from build123d import *

# Parameters (mm, degrees)
F0_R     = 7
F1_DEPTH = 25.4
F2_R     = 3.81
F3_DEPTH = 21.59
F4_R     = 7
F4_R_2   = 5.715
F5_DEPTH = 20.32
F6_W     = 2.794
F6_H     = 2.54
F7_DEPTH = 25.4
F8_R     = 0.9525
F9_DEPTH = 5.08


with BuildPart() as f1:
    # F0 (on Top) → F1 (new body)
    with BuildSketch(Plane.XY):
        Circle(F0_R)
    extrude(amount=F1_DEPTH)

    # F2 (on face) → F3 (cut)
    with BuildSketch(Plane.XY.offset(25.4)):
        Circle(F2_R)
    extrude(amount=-F3_DEPTH, mode=Mode.SUBTRACT)

    # F4 (on face) → F5 (cut)
    with BuildSketch(Plane(origin=(0, 0, 0), x_dir=(1, 0, 0), z_dir=(0, 0, -1))):
        Circle(F4_R)
        Circle(F4_R_2, mode=Mode.SUBTRACT)
    extrude(amount=-F5_DEPTH, mode=Mode.SUBTRACT)

    # F6 (on face) → F7 (cut)
    with BuildSketch(Plane(origin=(0, 0, 20.32), x_dir=(1, 0, 0), z_dir=(0, 0, -1))):
        with Locations((6.969102, 0)):
            Rectangle(F6_W, F6_H)
        with Locations((-6.969102, 0)):
            Rectangle(F6_W, F6_H)
    extrude(amount=-F7_DEPTH, mode=Mode.SUBTRACT)

    # F8 (on face) → F9 (join)
    with BuildSketch(Plane.XY.offset(3.81)):
        Circle(F8_R)
    extrude(amount=F9_DEPTH)


solid = f1.part
Design review of the part built by this model. Coordinates are the model's own, in mm. A direction names the side the tool comes from. Round coordinates to 2 decimals unless told otherwise and drop trailing zeros. Write each loop counter-clockwise with the first axis right and the second up, starting at its lowest first coordinate (ties: lowest second). Pieces come first, ordered by that corner, then holes. Notation, with made-up numbers: (76, -12.75) -> (101, -12.75) arc R34 cw to (101, 18.25) -> close; hole circle Ø11 at (-4, 85). An arc over 180 degrees is marked (long way). One line per item, written item: value. Start each with the question number.
Q1. The part is to be moulded in two halves that separate along Y. For faces 1 (the face through (6, 1.27, 23)), 2 (the face through (1, -1, 3.81)), 3 (the face through (0, 0, 0)), 4 (the face through (0, 7, 23)), say which applies: pulls with the +Y half, pulls with the -Y half, needs draft (parallel to the pull), parting line crosses it, or undercut.
Q2. To check wall thickness, follow probe 1 along Y at (x, z) = (0, 19.5) (3 decimals); probe 2 along Z at (x, y) = (-3, 5); probe 3 along Z at (x, y) = (1.5, 3). State the ranges of each line that lie inside material, in increasing order.
Q3. Add section C-C (x = 0). Give the boundary of the cut face in (y, z) (1 decimal), then the cut area to 3 significant figures.
Q4. Add section B-B (z = 23.5). Give the boundary of the cut face in (x, y), then the cut area to 3 significant figures.
Q5. Insertion check: P1, Ø6, axis at y = 2.5, z = 21, coming from the -X side; P2, Ø3, axis at y = 1, z = 5, coming from the -X side (3 decimals); P3, Ø0.8, axis at y = 0.5, z = 24, coming from the -X side; P4, Ø6, axis at x = 5, z = 6.5, coming from the -Y side. Each pin has a flat end and moves straight along its axis. Give the tip position at first contact, or say it passes through.
Q6. Add section D-D (y = -1.75). Give the boundary of the cut face in (x, z).
Q7. Tool access review of faces 5 (the face through (-0.83, -3.72, 14.76)), 6 (the face through (5.45, -1.72, 10.02)), 7 (the face through (-1, 6, 20.32)), 8 (the face through (-5.572, 0, 23)): name each direction out of +Z, -Z, +X, -X, +Y, -Y from which nothing blocks a thin tool from reaching the whole face with its end or side.
Response:
1. face 1: undercut
1. face 2: undercut
1. face 3: needs draft
1. face 4: pulls with the +Y half
2. probe 1: y = -5.715 to -3.81, 3.81 to 5.715
2. probe 2: z = 20.32 to 25.4
2. probe 3: z = 0 to 3.81
3. outline: (-7, 20.3) -> (-5.7, 20.3) -> (-5.7, 0) -> (5.7, 0) -> (5.7, 20.3) -> (7, 20.3) -> (7, 25.4) -> (3.8, 25.4) -> (3.8, 3.8) -> (1, 3.8) -> (1, 8.9) -> (-1, 8.9) -> (-1, 3.8) -> (-3.8, 3.8) -> (-3.8, 25.4) -> (-7, 25.4) -> close
3. area: 149 mm^2
4. outline: (-6.88, -1.27) arc R7 ccw to (6.88, -1.27) -> (5.57, -1.27) -> (5.57, 1.27) -> (6.88, 1.27) arc R7 ccw to (-6.88, 1.27) -> (-5.57, 1.27) -> (-5.57, -1.27) -> close; hole circle Ø7.62 at (0, 0)
4. area: 101 mm^2
5. P1: stops at x = -6.88
5. P2: stops at x = -5.715
5. P3: stops at x = -5.57
5. P4: stops at y = -5.35
6. outline: (-6.78, 20.32) -> (-5.44, 20.32) -> (-5.44, 0) -> (5.44, 0) -> (5.44, 20.32) -> (6.78, 20.32) -> (6.78, 25.4) -> (3.38, 25.4) -> (3.38, 3.81) -> (-3.38, 3.81) -> (-3.38, 25.4) -> (-6.78, 25.4) -> close
7. face 5: +Z
7. face 6: -Z
7. face 7: -Z, +Y
7. face 8: +Z, -X
